from build123d import *

# Parameters (mm, degrees)
SKETCH1_R           = 0.65
SKETCH1_R_2         = 0.785
BOSS_EXTRUDE1_DEPTH = 0.5
FILLET1_R           = 0.5
SKETCH6_R           = 1.426206797
BOSS_EXTRUDE3_DEPTH = 1.44
CHAMFER1_SIZE       = 1.4


with BuildPart() as part:
    # Sketch1 → Boss-Extrude1 (new body)
    with BuildSketch(Plane.XY):
        Polygon((0, 0), (9.19, 0), (9.19, -10.3886), (6.095, -10.3886), (6.095, -16.99), (3.095, -16.99), (3.095, -10.3886), (0, -10.3886), align=None)
        with Locations((4.595, -15.49)):
            Circle(SKETCH1_R, mode=Mode.SUBTRACT)
        with Locations((4.595, -9.5786)):
            Circle(SKETCH1_R_2, mode=Mode.SUBTRACT)
    extrude(amount=BOSS_EXTRUDE1_DEPTH)

    # Fillet1
    fillet1_edges = [part.edges().sort_by_distance(p)[0] for p in [
        (0, 0, 0.25),
        (9.19, 0, 0.25),
        (9.19, -10.3886, 0.25),
        (6.095, -16.99, 0.25),
        (3.095, -16.99, 0.25),
        (0, -10.3886, 0.25),
    ]]
    fillet(fillet1_edges, radius=FILLET1_R)

    # Sketch6 → Boss-Extrude3 (add)
    with BuildSketch(Plane.XY.offset(0.5)):
        with Locations(Location((4.595, -5.1943, 0), (0, 0, 180))):
            Circle(SKETCH6_R)
    extrude(amount=BOSS_EXTRUDE3_DEPTH)

    # Chamfer1
    chamfer1_edges = [part.edges().sort_by_distance(p)[0] for p in [
        (6.021206797, -5.1943, 0.5),
    ]]
    chamfer(chamfer1_edges, length=CHAMFER1_SIZE)


solid = part.part
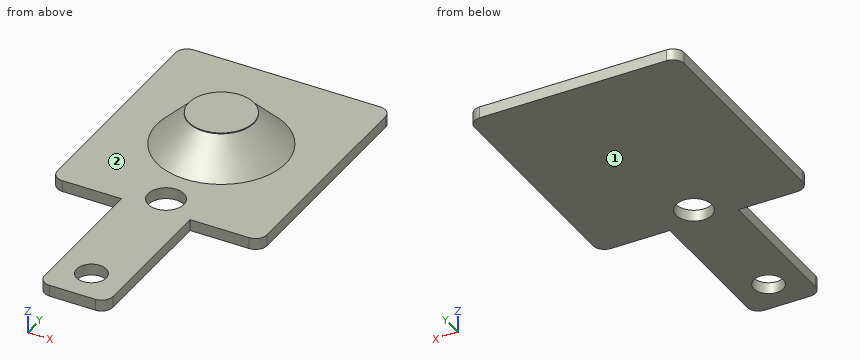
CAD build for the part. Positions are in the model's coordinates, mm. Face numbers are marked on the shaded views. A direction names the side the tool comes from. Coordinates: 2 decimals unless noted, no trailing zeros. Loops run counter-clockwise (first coordinate to the right, second up) from the corner with the lowest first, then second, coordinate; pieces in that order, holes last. Notation, with made-up numbers: (13, 49.25) - (68, 49.25) arc R20 ccw to (68, 68.25) - close; hole circle Ø4 at (-18.5, 77.5). An arc over 180 degrees is marked (long way). Write item = value, one per line. Start each with the question number.
Q1. Cut at A-A, the plane y = -15.49. List the corners of the cut face in (x, z) (3 decimals), then the cut area to 3 significant figures.
Q2. Cut at C-C, the plane y = -11.5. List the corners of the cut face in (x, z) (3 decimals).
Q3. Cut at B-B, the plane x = 0.75. List the corners of the cut face in (y, z).
Q4. Drill centre lines: L1, parallel to Y at x = 4.75, z = 0.25; L2, parallel to X at y = -15, z = 0.15 (3 decimals); L3, parallel to Z at x = 1.25, y = -2. Where is each one in solid material? Low to high.
Q5. Cut at D-D, the plane z = 1.1. List the corners of the cut face in (x, y) (3 decimals).
Q6. Which spindle directions (+Z, -Z, +X, -X, +Y, -Y) get a long thin tool onto all of the face, cutting with end or side? Do the marked faces 1 and 2. Say none if no direction does.
Computed:
q1.outline = (3.095, 0) - (3.945, 0) - (3.945, 0.5) - (3.095, 0.5) - close; (5.245, 0) - (6.095, 0) - (6.095, 0.5) - (5.245, 0.5) - close
q1.area = 0.850 mm²
q2.outline = (3.095, 0) - (6.095, 0) - (6.095, 0.5) - (3.095, 0.5) - close
q3.outline = (-10.39, 0) - (0, 0) - (0, 0.5) - (-10.39, 0.5) - close
q4.L1 = -16.99 to -16.12, -14.86 to -10.35, -8.81 to 0
q4.L2 = 3.095 to 4.168, 5.022 to 6.095
q4.L3 = 0 to 0.5
q5.outline = circle Ø4.452 at (4.595, -5.194)
q6.face_1 = -Z, +X, -X, +Y, -Y
q6.face_2 = +Z
